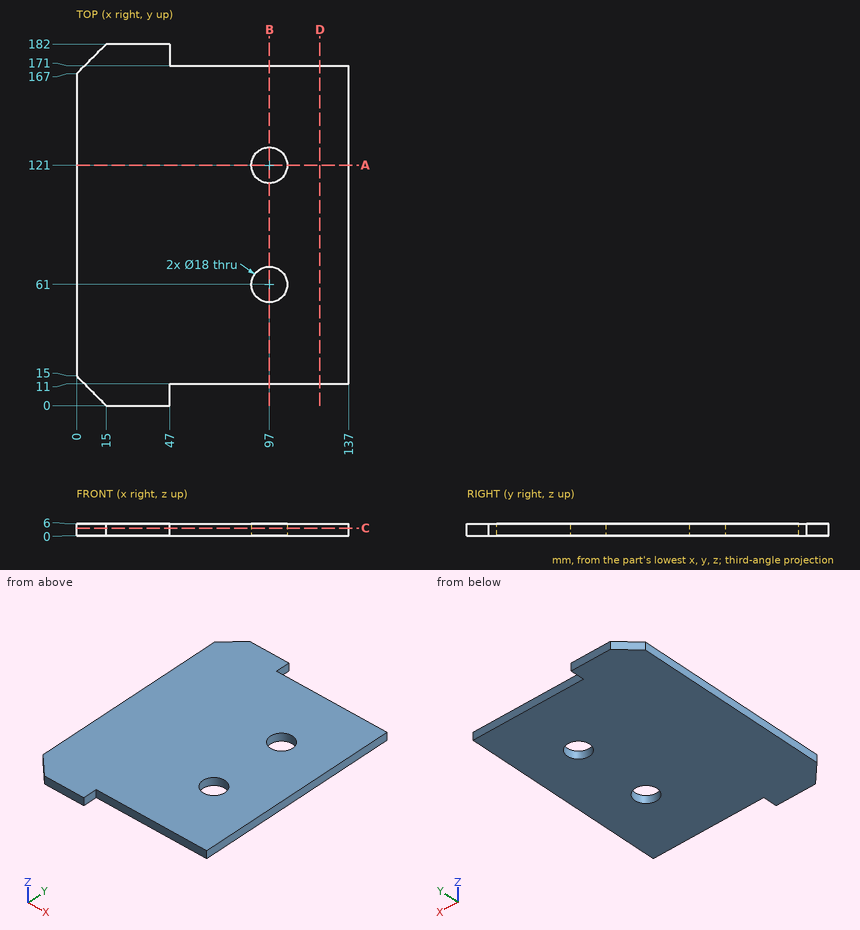
Drawing for the job (mm, zero at the part's lowest x, y, z). Give positions to 0.01 mm unless a question says otherwise; leave off trailing zeros. Write each loop counter-clockwise with the first axis right and the second up, starting at its lowest first coordinate (ties: lowest second). Pieces come first, ordered by that corner, then holes. Notation, with made-up numbers: M 56.5,74 L 95.5,74 A25 cw 95.5,113 Z; hole C 37,43 d2. An arc over 180 degrees is marked long. Return JSON: item names as keys, results as strings. Group by question number.
(1) Band-saw the part on A-A (y = 121). Give the cut face in (x, z), and give its area (3 significant figures).
(2) Band-saw the part on D-D (x = 122.5). Give the cut face in (y, z).
(3) Drill centre lines: L1, parallel to Y at x = 97, z = 3.5; L2, parallel to X at y = 61, z = 1.9; L3, parallel to Y at x = 105, z = 1. Where is each one in solid material? Low to high. Write a range as [from, to].
(4) Band-saw the part on B-B (x = 97). Give the cut face in (y, z).
(5) Band-saw the part on C-C (z = 3.75). Give the cut face in (x, y), and give its area (3 significant figures).
(6) Flat gauge pins, fed straight in: pin 1 Ø3 at (x, z) = (98.5, 3.5) entering from -Y; pin 2 Ø1 at (x, z) = (87.5, 3.5) entering from +Y; pin 3 Ø14.5 at (x, y) = (97, 121) entering from +Z; pin 4 Ø1.8 at (y, z) = (176.5, 2.5) entering from +X. Where does each tip first touch, or does it go through?
Entries:
{
 "1": {"outline": "M 0,0 L 88,0 L 88,6 L 0,6 Z; M 106,0 L 137,0 L 137,6 L 106,6 Z", "area": "714 mm^2"},
 "2": {"outline": "M 11,0 L 171,0 L 171,6 L 11,6 Z"},
 "3": {"L1": "y = [11, 52], [70, 112], [130, 171]", "L2": "x = [0, 88], [106, 137]", "L3": "y = [11, 56.88], [65.12, 116.88], [125.12, 171]"},
 "4": {"outline": "M 11,0 L 52,0 L 52,6 L 11,6 Z; M 70,0 L 112,0 L 112,6 L 70,6 Z; M 130,0 L 171,0 L 171,6 L 130,6 Z"},
 "5": {"outline": "M 0,15 L 15,0 L 47,0 L 47,11 L 137,11 L 137,171 L 47,171 L 47,182 L 15,182 L 0,167 Z; hole C 97,61 d18; hole C 97,121 d18", "area": "22,200 mm^2"},
 "6": {"pin 1": "stops at y = 11", "pin 2": "stops at y = 171", "pin 3": "passes through", "pin 4": "stops at x = 47"}
}
